Autodesk Inventor part; units mm, degrees
ref_plane "YZ Plane" through (0, 0, 0) normal (1, 0, 0) x (0, 1, 0)
ref_plane "XZ Plane" through (0, 0, 0) normal (0, 1, 0) x (-1, 0, 0)
ref_plane "XY Plane" through (0, 0, 0) normal (0, 0, 1) x (1, 0, 0)
sketch "Sketch1" plane through (0, 0, 0) normal (0, 0, 1) x (1, 0, 0)
  line L0 (0, 0) -> (243.149, 0)
  line L1 (243.149, 0) -> (243.149, 500)
  line L2 (243.149, 500) -> (0, 500)
  line L3 (0, 500) -> (0, 0)
  dimension "d0" = 243.149
  dimension "d1" = 500
extrude "Extrusion1" add sketch "Sketch1" along normal blind 18
sketch "Sketch2" plane through (0, 0, 0) normal (0, 0, -1) x (-1, 0, 0)
  line L0 (0, 0) -> (-243.149, 0)
  line L1 (-243.149, 500) -> (-235.149, 500)
  line L2 (-235.149, 500) -> (-235.149, 0)
  line L3 (-235.149, 0) -> (-243.149, 0)
  line L4 (-243.149, 0) -> (-243.149, 500)
  dimension "d4" = 8
extrude "Extrusion2" cut sketch "Sketch2" against normal blind 8
sketch "Sketch4" plane through (0, 500, 18) normal (0, 1, 0) x (1, 0, 0)
  line L0 (0, 18) -> (0, 0)
  line L1 (243.149, 0) -> (0, 0)
  line L2 (0, 0) -> (3.1489, 0)
  line L3 (0, 18) -> (0, 0)
  line L4 (3.1489, 0) -> (0, 18)
  dimension "d11" = 9.923
extrude "Extrusion4" cut sketch "Sketch4" against normal up to next
properties part number "regalboden"
Geometry: final body of the model. Coordinates: model frame, mm. Give positions to 0.01 mm unless a question says otherwise; leave off trailing zeros. Write each loop counter-clockwise with the first axis right and the second up, starting at its lowest first coordinate (ties: lowest second). Pieces come first, ordered by that corner, then holes.
1. Line query: probe 1 along X at (y, z) = (156, 11); probe 2 along X at (y, z) = (444.5, 12.5). Output: solid intervals per line, ascending.
2. Pin query (flat end, axial travel): P1, Ø5, axis at y = 246.5, z = 8.5, coming from the -X side; P2, Ø12, axis at x = 189, y = 265, coming from the -Z side; P3, Ø6, axis at y = 153.5, z = 14.5, coming from the -X side; P4, Ø9, axis at x = 240.5, y = 163.5, coming from the -Z side. Return the tip coordinate at first contact, or that it passes through.
3. Section query A-A, the plane y = 450. Return loops of the section in (x, z).
Computed:
1. probe 1: x = 1.92 to 243.15
1. probe 2: x = 2.19 to 243.15
2. P1: stops at x = 1.05
2. P2: stops at z = 0
2. P3: stops at x = 2.01
2. P4: stops at z = 8
3. outline: (0, 0) - (235.15, 0) - (235.15, 8) - (243.15, 8) - (243.15, 18) - (3.15, 18) - close
